```python
from build123d import *

# Parameters (mm, degrees)
F1_DEPTH = 63.5
F2_DEPTH = 25.4
F3_DEPTH = 7.9375
F0_W     = 25.6498904824
F0_H     = 19.05
F4_DEPTH = 25.4
F6_R     = 6.35


with BuildPart() as f1:
    # F0 (on Front) → F1 (new body, symmetric)
    with BuildSketch(Plane.XZ):
        Polygon((41.275, -9.525), (41.275, 9.525), (22.225, 9.525), (-41.275, 9.525), (-41.275, -9.525), align=None)
    extrude(amount=F1_DEPTH, both=True)

    # F0 (on Front) → F2 (join, symmetric)
    with BuildSketch(Plane.XZ):
        with BuildLine():
            Line((22.225, 9.525), (41.275, 9.525))
            Line((41.275, 9.525), (41.275, 27.0002))
            ThreePointArc((41.275, 27.0002), (45.9246798487, 38.2255201513), (57.15, 42.8752))
            Line((57.15, 42.8752), (60.0751095176, 42.8752))
            Line((60.0751095176, 42.8752), (60.0751095176, 61.9252))
            Line((60.0751095176, 61.9252), (57.15, 61.9252))
            add(Edge.make_bspline(
                [(57.15, 61.9252), (56.3562246921, 61.9012944132), (55.5537204814, 61.8737200554), (54.7431620422, 61.8421683147)],
                knots=[0, 0, 0, 0, 2.5014710885, 2.5014710885, 2.5014710885, 2.5014710885], degree=3))
            ThreePointArc((54.7431620422, 61.8421683147), (31.617526161, 50.8297699639), (22.225, 27.0002))
            Line((22.225, 27.0002), (22.225, 9.525))
        make_face()
    extrude(amount=F2_DEPTH, both=True)

    # F0 (on Front) → F3 (join, symmetric)
    with BuildSketch(Plane.XZ):
        with BuildLine():
            Line((-41.275, 9.525), (22.225, 9.525))
            Line((22.225, 9.525), (22.225, 27.0002))
            ThreePointArc((22.225, 27.0002), (31.617526161, 50.8297699639), (54.7431620422, 61.8421683147))
            add(Edge.make_bspline(
                [(54.7431620422, 61.8421683147), (19.4226041922, 60.4672827696), (-31.1915768934, 51.5400171012), (-41.275, 9.525)],
                knots=[2.5014710885, 2.5014710885, 2.5014710885, 2.5014710885, 111.5045361635, 111.5045361635, 111.5045361635, 111.5045361635], degree=3))
        make_face()
    extrude(amount=F3_DEPTH, both=True)

    # F0 (on Front) → F4 (join, symmetric)
    with BuildSketch(Plane.XZ):
        with Locations((72.9000547588, 52.4002)):
            Rectangle(F0_W, F0_H)
    extrude(amount=F4_DEPTH, both=True)

    # F0 (on Front) → F5 (revolve)
    with BuildSketch(Plane.XZ):
        Polygon((85.725, 61.9252), (85.725, 42.8752), (85.725, 38.1), (110.8751095176, 38.1), (110.8751095176, 66.675), (85.725, 66.675), align=None)
    revolve(axis=Axis((85.725, 0, 52.3875), (0, 0, -1)))

    # F6
    f6_edges = [f1.edges().sort_by_distance(p)[0] for p in [
        (41.275, -63.5, 0),
        (-41.275, -63.5, 0),
        (41.275, 63.5, 0),
        (-41.275, 63.5, 0),
    ]]
    fillet(f6_edges, radius=F6_R)


solid = f1.part
```
Read the model definition and answer for the solid it produces. Units are mm, in the model's axes. A direction names the side the tool comes from. Coordinates: 2 decimals unless noted, no trailing zeros. Loops run counter-clockwise (first coordinate to the right, second up) from the corner with the lowest first, then second, coordinate; pieces in that order, holes last. Notation, with made-up numbers: (-25.5, 38) - (2.5, 38) arc R31 ccw to (2.5, 76) - close; hole circle Ø4 at (-35.5, -1.75). An arc over 180 degrees is marked (long way). Answer in a Markdown table with one row per item.
1. Which of the six approach directions +Z, -Z, +X, -X, +Y, -Y give full straight-line access (tool end or side, diameter ignored) to faces 1 (the face through (41.275, -1, 4)), 2 (the face through (46, 25.4, 42)), 3 (the face through (31.87, -16.79, 51.1))?
Conclusion:
| item | result |
|---|---|
| face 1 | -Z, +X, +Y, -Y |
| face 2 | +Z, +X, -X, +Y |
| face 3 | +Z, -X, -Y |
2. Find section A-A, the plane y = 54. Write down the section's boundary in (x, z) (3 decimals), then the cut area to 3 significant figures.
Conclusion:
| item | result |
|---|---|
| outline | (-41.275, -9.525) - (41.275, -9.525) - (41.275, 9.525) - (-41.275, 9.525) - close |
| area | 1,570 mm² |
3. Given pin 1 (4 mm diameter, centred on x = 81.5, z = 52, fed in from +Y); pin 2 (1 mm diameter, centred on y = -26.5, z = 44.5, fed in from +X); pin 3 (11 mm diameter, centred on y = 2, z = 12, fed in from +X) (3 decimals); pin 4 (8.5 mm diameter, centred on y = -20.5, z = 22.5, fed in from -X) (3 decimals), each flat-ended and moving along its own axis, determine where each tip first touches the part or whether it passes through.
Conclusion:
| item | result |
|---|---|
| pin 1 | stops at y = 25.4 |
| pin 2 | passes through |
| pin 3 | stops at x = 41.275 |
| pin 4 | stops at x = 22.225 |
4. Straight lines are drawn through the part: line 1 (Z direction, x = -33, y = 36) (3 decimals); line 2 (Y direction, x = 49, z = 56.5); line 3 (X direction, y = 19, z = 15.5) (3 decimals). For each, find the intervals that lie inside material, in ascending order.
Conclusion:
| item | result |
|---|---|
| line 1 | z = -9.525 to 9.525 |
| line 2 | y = -25.4 to 25.4 |
| line 3 | x = 22.225 to 41.275 |
5. Determine the mould class of faces 4 (the face through (-1, -1, -9.525)), 5 (the face through (-41.275, -1, 0)), 6 (the face through (60, 2, 42.875)) for opening direction X: +X half, -X half, draft (parallel to the pull), parting line (faces both ways), or undercut.
Conclusion:
| item | result |
|---|---|
| face 4 | draft |
| face 5 | -X half |
| face 6 | undercut |
